Drawing for the job (mm, zero at the part's lowest x, y, z). Give positions to 0.01 mm unless a question says otherwise; leave off trailing zeros. Loops run counter-clockwise (first coordinate to the right, second up) from the corner with the lowest first, then second, coordinate; pieces in that order, holes last. Notation, with made-up numbers: (-8, -4.5) - (48, -4.5) arc R36 ccw to (48, 33.5) - close; hole circle Ø5 at (88.25, 81.25). An arc over 180 degrees is marked (long way). Return JSON: item names as keys, results as strings. Group by question number.
1) Slice it at C-C (z = 320.5). List the corners of the cut face in (x, y).
2) Drop flat-ended pins along their axis: pin 1 (5 mm diameter, centred on x = 44.5, y = 88, fed in from -Z); pin 2 (8 mm diameter, centred on x = 259.49, y = 16.92, fed in from +Z); pin 3 (4 mm diameter, centred on y = 236.5, z = 351, fed in from +X). Give the stop position or say it passes through.
3) Drill centre lines: probe 1 along Y at (x, z) = (200, 445.5); probe 2 along X at (y, z) = (205, 420.5); probe 3 along Y at (x, z) = (194, 380.5). Where is each one in solid material? Low to high. Write a range as from..to.
4) Mould opens along Y. For the marked faces 1 and 2 say: released by +Y, released by -Y, zero draft, split by the parting line, or undercut.
5) Slice it at B-B (y = 272.5). List the corners of the cut face in (x, z).
6) Slice it at A-A (x = 200). List the corners of the cut face in (y, z), and give its area (3 significant figures).
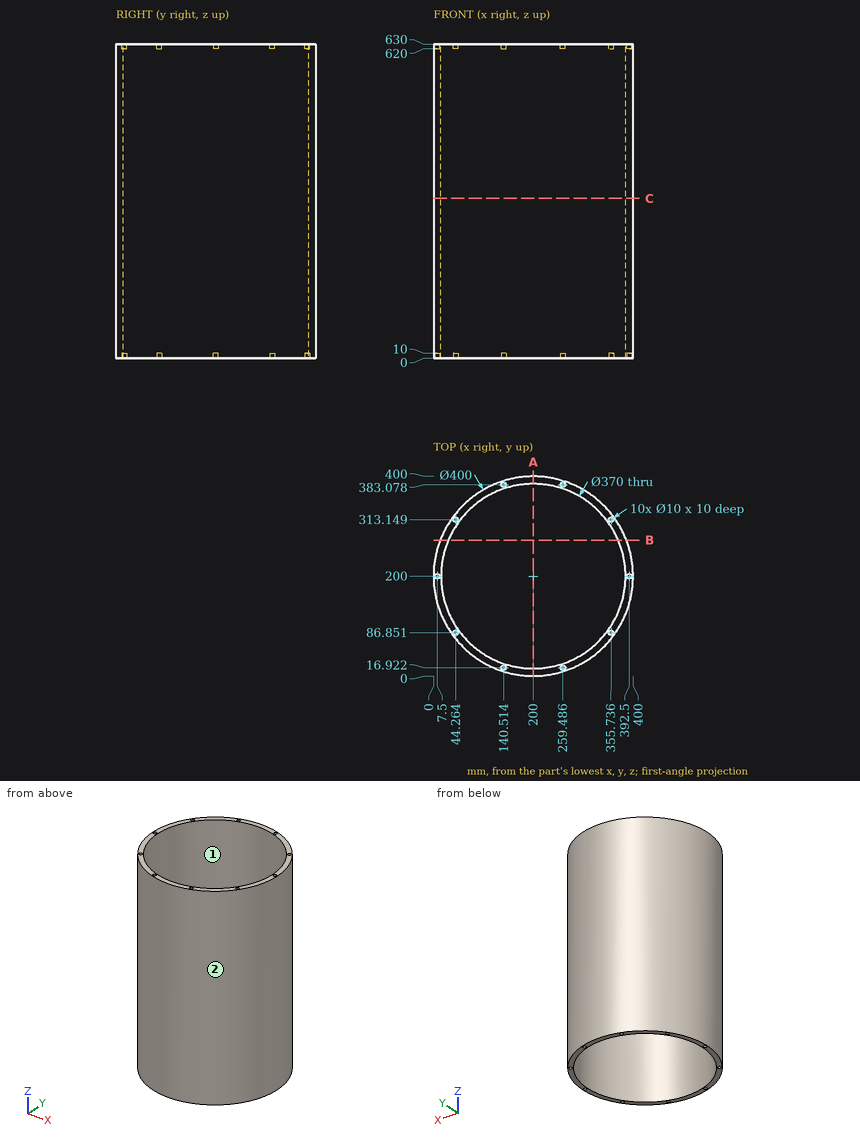
Results:
{
 "1": {"outline": "circle Ø400 at (200, 200); hole circle Ø370 at (200, 200)"},
 "2": {"pin 1": "z = 10", "pin 2": "z = 620", "pin 3": "x = 397"},
 "3": {"probe 1": "0..15, 385..400", "probe 2": "0.06..15.07, 384.93..399.94", "probe 3": "0.09..15.1, 384.9..399.91"},
 "4": {"face 1": "undercut", "face 2": "split by the parting line"},
 "5": {"outline": "(13.6, 0) - (29.8, 0) - (29.8, 630) - (13.6, 630) - close; (370.2, 0) - (386.4, 0) - (386.4, 630) - (370.2, 630) - close"},
 "6": {"outline": "(0, 0) - (15, 0) - (15, 630) - (0, 630) - close; (385, 0) - (400, 0) - (400, 630) - (385, 630) - close", "area": "18,900 mm2"}
}
